from build123d import *

# Parameters (mm, degrees)
SKETCH1_R           = 34.5
SKETCH1_R_2         = 1.5635
SKETCH1_R_3         = 7.4
BOSS_EXTRUDE1_DEPTH = 1
BOSS_EXTRUDE2_START = 14.2875
SKETCH1_3_R         = 27.69
SKETCH1_3_R_2       = 7.4
SKETCH1_3_R_3       = 1.5635
BOSS_EXTRUDE2_DEPTH = 14.2875
SKETCH2_R           = 3
SKETCH2_R_2         = 1.5635
CUT_EXTRUDE1_DEPTH  = 4.7625
CUT_EXTRUDE4_START  = -1
CUT_EXTRUDE4_DEPTH  = 4.7625


with BuildPart() as part:
    # Sketch1 → Boss-Extrude1 (new body)
    with BuildSketch(Plane(origin=(0, 0, 0), x_dir=(1, 0, 0), z_dir=(0, 1, 0))):
        with Locations(Location((0, 0, 0), (0, 0, 270))):
            Circle(SKETCH1_R)
        with Locations(Location((22.5, 0, 0), (0, 0, 270))):
            Circle(SKETCH1_R_2, mode=Mode.SUBTRACT)
        with Locations(Location((15.909902577, -15.909902577, 0), (0, 0, 270))):
            Circle(SKETCH1_R_2, mode=Mode.SUBTRACT)
        with Locations(Location((0, -22.5, 0), (0, 0, 270))):
            Circle(SKETCH1_R_2, mode=Mode.SUBTRACT)
        with Locations(Location((-15.909902577, -15.909902577, 0), (0, 0, 270))):
            Circle(SKETCH1_R_2, mode=Mode.SUBTRACT)
        with Locations(Location((-22.5, 0, 0), (0, 0, 270))):
            Circle(SKETCH1_R_2, mode=Mode.SUBTRACT)
        with Locations(Location((-15.909902577, 15.909902577, 0), (0, 0, 270))):
            Circle(SKETCH1_R_2, mode=Mode.SUBTRACT)
        with Locations(Location((0, 22.5, 0), (0, 0, 270))):
            Circle(SKETCH1_R_2, mode=Mode.SUBTRACT)
        with Locations(Location((15.909902577, 15.909902577, 0), (0, 0, 270))):
            Circle(SKETCH1_R_2, mode=Mode.SUBTRACT)
        with Locations(Location((0, 0, 0), (0, 0, 270))):
            Circle(SKETCH1_R_3, mode=Mode.SUBTRACT)
    extrude(amount=-BOSS_EXTRUDE1_DEPTH)

    # Sketch1_3 → Boss-Extrude2 (add)
    with BuildSketch(Plane(origin=(0, 0, 0), x_dir=(1, 0, 0), z_dir=(0, 1, 0)).offset(BOSS_EXTRUDE2_START)):
        with Locations(Location((0, 0, 0), (0, 0, 270))):
            Circle(SKETCH1_3_R)
        with Locations(Location((0, 0, 0), (0, 0, 270))):
            Circle(SKETCH1_3_R_2, mode=Mode.SUBTRACT)
        with Locations(Location((-15.909902577, -15.909902577, 0), (0, 0, 270))):
            Circle(SKETCH1_3_R_3, mode=Mode.SUBTRACT)
        with Locations(Location((0, -22.5, 0), (0, 0, 270))):
            Circle(SKETCH1_3_R_3, mode=Mode.SUBTRACT)
        with Locations(Location((15.909902577, -15.909902577, 0), (0, 0, 270))):
            Circle(SKETCH1_3_R_3, mode=Mode.SUBTRACT)
        with Locations(Location((-22.5, 0, 0), (0, 0, 270))):
            Circle(SKETCH1_3_R_3, mode=Mode.SUBTRACT)
        with Locations(Location((-15.909902577, 15.909902577, 0), (0, 0, 270))):
            Circle(SKETCH1_3_R_3, mode=Mode.SUBTRACT)
        with Locations(Location((0, 22.5, 0), (0, 0, 270))):
            Circle(SKETCH1_3_R_3, mode=Mode.SUBTRACT)
        with Locations(Location((22.5, 0, 0), (0, 0, 270))):
            Circle(SKETCH1_3_R_3, mode=Mode.SUBTRACT)
        with Locations(Location((15.909902577, 15.909902577, 0), (0, 0, 270))):
            Circle(SKETCH1_3_R_3, mode=Mode.SUBTRACT)
    extrude(amount=-BOSS_EXTRUDE2_DEPTH)

    # Sketch2 → Cut-Extrude1 (cut)
    # profile 1 of 4: a face of its own
    with BuildSketch(Plane(origin=(0, 14.2875, 0), x_dir=(1, 0, 0), z_dir=(0, 1, 0))):
        with Locations(Location((-15.909902577, 15.909902577, 0), (0, 0, 270))):
            Circle(SKETCH2_R)
        with Locations(Location((-15.909902577, 15.909902577, 0), (0, 0, 270))):
            Circle(SKETCH2_R_2, mode=Mode.SUBTRACT)
    # profile 2 of 4: a face of its own
    with BuildSketch(Plane(origin=(0, 14.2875, 0), x_dir=(1, 0, 0), z_dir=(0, 1, 0))):
        with Locations(Location((15.909902577, 15.909902577, 0), (0, 0, 270))):
            Circle(SKETCH2_R)
        with Locations(Location((15.909902577, 15.909902577, 0), (0, 0, 270))):
            Circle(SKETCH2_R_2, mode=Mode.SUBTRACT)
    # profile 3 of 4: a face of its own
    with BuildSketch(Plane(origin=(0, 14.2875, 0), x_dir=(1, 0, 0), z_dir=(0, 1, 0))):
        with Locations(Location((-15.909902577, -15.909902577, 0), (0, 0, 270))):
            Circle(SKETCH2_R)
        with Locations(Location((-15.909902577, -15.909902577, 0), (0, 0, 270))):
            Circle(SKETCH2_R_2, mode=Mode.SUBTRACT)
    # profile 4 of 4: a face of its own
    with BuildSketch(Plane(origin=(0, 14.2875, 0), x_dir=(1, 0, 0), z_dir=(0, 1, 0))):
        with Locations(Location((15.909902577, -15.909902577, 0), (0, 0, 270))):
            Circle(SKETCH2_R)
    extrude(amount=-CUT_EXTRUDE1_DEPTH, mode=Mode.SUBTRACT)

    # Sketch4 → Cut-Extrude4 (cut)
    with BuildSketch(Plane.XZ.offset(1).offset(CUT_EXTRUDE4_START)):
        Polygon((22.5, 3.117691454), (19.8, 1.558845727), (19.8, -1.558845727), (22.5, -3.117691454), (25.2, -1.558845727), (25.2, 1.558845727), align=None)
        Polygon((1.558845727, 25.2), (-1.558845727, 25.2), (-3.117691454, 22.5), (-1.558845727, 19.8), (1.558845727, 19.8), (3.117691454, 22.5), align=None)
        Polygon((3.117691454, -22.5), (1.558845727, -19.8), (-1.558845727, -19.8), (-3.117691454, -22.5), (-1.558845727, -25.2), (1.558845727, -25.2), align=None)
        Polygon((-22.5, -3.117691454), (-19.8, -1.558845727), (-19.8, 1.558845727), (-22.5, 3.117691454), (-25.2, 1.558845727), (-25.2, -1.558845727), align=None)
    extrude(amount=-CUT_EXTRUDE4_DEPTH, mode=Mode.SUBTRACT)


solid = part.part
Read the model definition and answer for the solid it produces. Units are mm, in the model's axes. A direction names the side the tool comes from. Give positions to 0.01 mm unless a question says otherwise; leave off trailing zeros. Write each loop counter-clockwise with the first axis right and the second up, starting at its lowest first coordinate (ties: lowest second). Pieces come first, ordered by that corner, then holes. Notation, with made-up numbers: (9.5, 36.5) - (42.5, 36.5) arc R20 ccw to (42.5, 64.5) - close; hole circle Ø9 at (-5, -3). An arc over 180 degrees is marked (long way). Use CSV: the item, a comma, the result in double quotes. Start each with the question number.
Item 1: Flat-ended cylindrical pins translate along their axes: P1, Ø1.6, axis at x = -1, z = -23, coming from the +Y side; P2, Ø0.9, axis at x = 0.5, y = 2.5, coming from the +Z side; P3, Ø1, axis at x = 7, y = 10, coming from the -Z side; P4, Ø0.9, axis at x = 0, y = 1.5, coming from the -Z side. Find the tip coordinate at first contact, or state that the pin passes through.
Item 2: Consider line 1 (Z direction, x = 1.5, y = 3.75); line 2 (X direction, y = 3, z = 16); line 3 (X direction, y = 0.5, z = 21.5). Determine where each line is inside the solid, lowest interval first.
Item 3: The part is cut by section C-C, the plane z = 4. Give the vertices of the cut face in (x, y).
Item 4: The mould has two halves that part along X. Classify faces 4 (the cylindrical face through (1.217, 7.244, -27.663)), 5 (the flat face through (-21.17, 2.35, -2.35)): pulls with the +X half, pulls with the -X half, needs draft (parallel to the pull), parting line crosses it, or undercut.
Item 5: The part is cut by section A-A, the plane x = 4.5. Give the vertices of the cut face in (y, z), and give its area (3 significant figures).
Item 6: The part is cut by section B-B, the plane y = 1.5. Count the separate pieces of the cut face and the enclosed holes in it, and give its area (3 significant figures).
Item 7: For faces 1 (the flat face through (0, 2, -19.8)), 2 (the cylindrical face through (17.94, 11.94, 13.7)), 3 (the cylindrical face through (-0.599, -0.493, 23.944)), determine the directions among +Z, -Z, +X, -X, +Y, -Y from which every point of the face is accessible in a straight line to the end or side of a thin tool.
Taken from the geometry:
1,P1,"y = 14.29"
1,P2,"z = 27.69"
1,P3,"z = -26.92"
1,P4,"z = -27.69"
2,line 1,"-27.65 to -25.2, -19.8 to -7.25, 7.25 to 19.8, 25.2 to 27.65"
2,line 2,"-22.6 to -17.47, -14.35 to 14.35, 17.47 to 22.6"
2,line 3,"-17.45 to -2.54, 2.54 to 17.45"
3,outline,"(-34.27, -1) - (-6.23, -1) - (-6.23, 14.29) - (-27.4, 14.29) - (-27.4, 0) - (-34.27, 0) - close; (6.23, -1) - (34.27, -1) - (34.27, 0) - (27.4, 0) - (27.4, 14.29) - (6.23, 14.29) - close"
4,face 4,"parting line crosses it"
4,face 5,"undercut"
5,outline,"(-1, -34.21) - (0, -34.21) - (0, -27.32) - (14.29, -27.32) - (14.29, -5.87) - (-1, -5.87) - close; (-1, 5.87) - (14.29, 5.87) - (14.29, 27.32) - (0, 27.32) - (0, 34.21) - (-1, 34.21) - close"
5,area,"670 mm2"
6,separate pieces,"1"
6,enclosed holes,"9"
6,area,"2,110 mm2"
7,face 1,"none"
7,face 2,"+Y"
7,face 3,"+Y, -Y"
